from build123d import *

# Parameters (mm, degrees)
SKETCH_1_R          = 1.5
EXTRUDE_1_DEPTH     = 3
CUT_EXTRUDE_1_DEPTH = 10
SKETCH_3_R          = 1.5
CUT_EXTRUDE_2_DEPTH = 10
SKETCH_4_R          = 1
SKETCH_4_W          = 12.5
SKETCH_4_H          = 22.5
EXTRUDE_2_DEPTH     = 3
SKETCH_5_R          = 1
CUT_EXTRUDE_3_DEPTH = 10
FILLET_1_R          = 10
CUT_EXTRUDE_4_DEPTH = 10
FILLET_2_R          = 5


with BuildPart() as part:
    # 草图1 → 凸台-拉伸1 (new body)
    with BuildSketch(Plane.XY):
        with BuildLine():
            Line((30, 65), (43.229490169, 55))
            ThreePointArc((43.229490169, 55), (24.322951332, 45.093216766), (10.332713198, 28.972583968))
            ThreePointArc((10.332713198, 28.972583968), (0, 23.037780053), (-10.332713198, 28.972583968))
            ThreePointArc((-10.332713198, 28.972583968), (-24.322951332, 45.093216766), (-43.229490169, 55))
            Line((-43.229490169, 55), (-30, 65))
            Line((-30, 65), (-30, 107))
            ThreePointArc((-30, 107), (-27.071067812, 114.071067812), (-20, 117))
            Line((-20, 117), (20, 117))
            ThreePointArc((20, 117), (27.071067812, 114.071067812), (30, 107))
            Line((30, 107), (30, 65))
        make_face()
        with Locations((-30, 60)):
            Circle(SKETCH_1_R, mode=Mode.SUBTRACT)
        with Locations((-8, 30)):
            Circle(SKETCH_1_R, mode=Mode.SUBTRACT)
        with Locations((8, 30)):
            Circle(SKETCH_1_R, mode=Mode.SUBTRACT)
        with Locations((30, 60)):
            Circle(SKETCH_1_R, mode=Mode.SUBTRACT)
    extrude(amount=EXTRUDE_1_DEPTH)

    # 草图2 → 切除-拉伸1 (cut)
    with BuildSketch(Plane(origin=(0, 0, 0), x_dir=(-1, 0, 0), z_dir=(0, 0, -1))):
        with BuildLine():
            Line((14.08407385, 34.61181483), (12.108970584, 36.269123252))
            ThreePointArc((12.108970584, 36.269123252), (11.739200084, 40.49561941), (15.965696242, 40.865389911))
            Line((15.965696242, 40.865389911), (17.940799508, 39.208081488))
            Line((17.940799508, 39.208081488), (18.60524138, 38.39769253))
            Line((18.60524138, 38.39769253), (14.816805035, 33.83995685))
            Line((14.816805035, 33.83995685), (14.08407385, 34.61181483))
        make_face()
        with BuildLine():
            Line((-18.60524138, 38.39769253), (-17.940799508, 39.208081488))
            Line((-17.940799508, 39.208081488), (-15.965696242, 40.865389911))
            ThreePointArc((-15.965696242, 40.865389911), (-11.739200084, 40.49561941), (-12.108970584, 36.269123252))
            Line((-12.108970584, 36.269123252), (-14.08407385, 34.61181483))
            Line((-14.08407385, 34.61181483), (-14.816805035, 33.83995685))
            Line((-14.816805035, 33.83995685), (-18.60524138, 38.39769253))
        make_face()
    extrude(amount=-CUT_EXTRUDE_1_DEPTH, mode=Mode.SUBTRACT)

    # 草图3 → 切除-拉伸2 (cut)
    with BuildSketch(Plane(origin=(0, 0, 0), x_dir=(-1, 0, 0), z_dir=(0, 0, -1))):
        with Locations((-25, 102)):
            Circle(SKETCH_3_R)
        with Locations((-25, 87)):
            Circle(SKETCH_3_R)
        with Locations((25, 102)):
            Circle(SKETCH_3_R)
        with Locations((25, 87)):
            Circle(SKETCH_3_R)
        with BuildLine():
            Line((-8.458896236, 64.355158964), (-8.458896236, 94.5))
            ThreePointArc((-8.458896236, 94.5), (0, 102.958896236), (8.458896236, 94.5))
            Line((8.458896236, 94.5), (8.458896236, 64.355158964))
            ThreePointArc((8.458896236, 64.355158964), (0, 55.896262728), (-8.458896236, 64.355158964))
        make_face()
    extrude(amount=-CUT_EXTRUDE_2_DEPTH, mode=Mode.SUBTRACT)

    # 草图4 → 凸台-拉伸2 (add)
    with BuildSketch(Plane(origin=(0, 0, 0), x_dir=(-1, 0, 0), z_dir=(0, 0, -1))):
        with BuildLine():
            Line((-9.51564662, 141.75), (-20, 117))
            Line((-20, 117), (-9.51564662, 117))
            Line((-9.51564662, 117), (-2.844735856, 108.972139798))
            Line((-2.844735856, 108.972139798), (9.51564662, 117))
            Line((9.51564662, 117), (20, 117))
            Line((20, 117), (9.51564662, 141.75))
            ThreePointArc((9.51564662, 141.75), (0, 151.26564662), (-9.51564662, 141.75))
        make_face()
        with Locations((0, 141.75)):
            Circle(SKETCH_4_R, mode=Mode.SUBTRACT)
        with Locations((0, 128.25)):
            Rectangle(SKETCH_4_W, SKETCH_4_H, mode=Mode.SUBTRACT)
    extrude(amount=-EXTRUDE_2_DEPTH)

    # 草图5 → 切除-拉伸3 (cut)
    with BuildSketch(Plane(origin=(0, 0, 0), x_dir=(-1, 0, 0), z_dir=(0, 0, -1))):
        with Locations((0, 114.75)):
            Circle(SKETCH_5_R)
    extrude(amount=-CUT_EXTRUDE_3_DEPTH, mode=Mode.SUBTRACT)

    # 圆角1
    fillet_1_edges = [part.edges().sort_by_distance(p)[0] for p in [
        (9.51564662, 141.75, 1.5),
        (-9.51564662, 141.75, 1.5),
        (-20, 117, 1.5),
        (20, 117, 1.5),
    ]]
    fillet(fillet_1_edges, radius=FILLET_1_R)

    # 草图6 → 切除-拉伸4 (cut)
    with BuildSketch(Plane(origin=(0, 0, 0), x_dir=(-1, 0, 0), z_dir=(0, 0, -1))):
        Polygon((-30, 107), (30, 107), (76.168650248, 160.022811959), (-16.915973461, 154.626601889), (-34.871476016, 113.990464525), align=None)
    extrude(amount=-CUT_EXTRUDE_4_DEPTH, mode=Mode.SUBTRACT)

    # 圆角2
    fillet_2_edges = [part.edges().sort_by_distance(p)[0] for p in [
        (30, 107, 1.5),
        (-30, 107, 1.5),
    ]]
    fillet(fillet_2_edges, radius=FILLET_2_R)


solid = part.part
Work out the finished part from the listing and answer in its coordinate system (mm). A direction names the side the tool comes from. Coordinates: 2 decimals unless noted, no trailing zeros. Write each loop counter-clockwise with the first axis right and the second up, starting at its lowest first coordinate (ties: lowest second). Pieces come first, ordered by that corner, then holes. Notation, with made-up numbers: M 54,5.25 L 58,5.25 A25 ccw 58,32.25 Z; hole C 46,-9.5 d1. An arc over 180 degrees is marked long. Answer as CSV lines item,"result". Start each with the question number.
Item 1: Section D-D on z = 1.3 is taken. Give the number of separate pieces and of enclosed holes in the cut face, and give its area (3 significant figures).
Item 2: Flat-ended cylindrical pins translate along their axes: P1, Ø1.5, axis at y = 75, z = 1.5, coming from the +X side; P2, Ø1, axis at y = 39, z = 1.5, coming from the +X side; P3, Ø1, axis at x = -23, z = 1.5, coming from the -Y side. Find the tip coordinate at first contact, or state that the pin passes through.
Item 3: Determine the mould class of faces 1 (the face through (0.186, 102.957, 1.479)), 2 (the face through (-8.459, 80, 1)), 3 (the face through (-30, 83, 1)), 4 (the face through (13.083, 35.452, 1.479)) for opening direction X: released by +X, released by -X, zero draft, split by the parting line, or undercut.
Item 4: Section A-A on y = 70.5 is taken. Write down the section's boundary in (x, z).
Item 5: Section C-C on x = -5.5 is taken. Write down the section's boundary in (y, z), and give its area (3 significant figures).
Item 6: Section B-B on y = 87 is taken. Write down the section's boundary in (x, z).
Item 7: A tool of negligible diameter and unlimited length cuts with its end or side. For faces 5 (the face through (17, 40, 1)), 6 (the face through (-13.11, 35.43, 1.48)), 7 (the face through (8.459, 79, 1)), 8 (the face through (30, 84, 1)), 9 (the face through (-9, 75, 0)), from which of +Z, -Z, +X, -X, +Y, -Y can it reach the whole face along a straight path? Write none if from no direction.
Item 8: Consider L1, parallel to X at y = 87, z = 0.85; L2, parallel to X at y = 74, z = 0.25; L3, parallel to X at y = 102, z = 0.95. Determine where each line is inside the solid, lowest interval first.
Checks:
1,separate pieces,"1"
1,enclosed holes,"9"
1,area,"3,650 mm²"
2,P1,"stops at x = 30"
2,P2,"stops at x = 18.21"
2,P3,"stops at y = 43.59"
3,face 1,"undercut"
3,face 2,"undercut"
3,face 3,"released by -X"
3,face 4,"released by +X"
4,outline,"M -30,0 L -8.46,0 L -8.46,3 L -30,3 Z; M 8.46,0 L 30,0 L 30,3 L 8.46,3 Z"
5,outline,"M 24.38,0 L 57.93,0 L 57.93,3 L 24.38,3 Z; M 100.93,0 L 107,0 L 107,3 L 100.93,3 Z"
5,area,"119 mm²"
6,outline,"M -30,0 L -26.5,0 L -26.5,3 L -30,3 Z; M -23.5,0 L -8.46,0 L -8.46,3 L -23.5,3 Z; M 8.46,0 L 23.5,0 L 23.5,3 L 8.46,3 Z; M 26.5,0 L 30,0 L 30,3 L 26.5,3 Z"
7,face 5,"+Z, -Z, -Y"
7,face 6,"+Z, -Z, -X"
7,face 7,"+Z, -Z"
7,face 8,"+Z, -Z, +X, +Y"
7,face 9,"-Z, +X, -X, +Y, -Y"
8,L1,"x = -30 to -26.5, -23.5 to -8.46, 8.46 to 23.5, 26.5 to 30"
8,L2,"x = -30 to -8.46, 8.46 to 30"
8,L3,"x = -30 to -26.5, -23.5 to -3.91, 3.91 to 23.5, 26.5 to 30"
